Autodesk Inventor part; units mm, degrees
ref_plane "Work Plane1" through (-11.0913, 6.35, -8.8477) normal (0, -0.4472, -0.8944) x (1, 0, 0)
ref_plane "Work Plane2" through (-7.9163, 6.35, -5.6727) normal (-0.8944, -0.4472, 0) x (0, 0, -1)
ref_plane "Work Plane3" through (-7.9163, 6.35, -5.6727) normal (-0.8944, 0.4472, 0) x (0, 0, -1)
sketch "Sketch1" plane through (0, 0, 0) normal (0, 1, 0) x (-1, 0, 0)
  line L0 (11.0913, -5.6727) -> (4.7413, -5.6727)
  line L1 (4.7413, -5.6727) -> (4.7413, -12.0227)
  line L2 (4.7413, -12.0227) -> (11.0913, -12.0227)
  line L3 (11.0913, -12.0227) -> (11.0913, -5.6727)
  point P0 (0, 0)
  dimension "d0" = 6.35
  dimension "d1" = 6.35
extrude "Extrusion1" add sketch "Sketch1" along normal blind 6.35
sketch "Sketch2" plane through (0, 6.35, 0) normal (0, 1, 0) x (1, 0, 0)
  line L0 (-11.0913, 5.6727) -> (-4.7413, 5.6727)
  line L1 (-7.9163, 5.6727) -> (-7.9163, 31.288)
  line L2 (-11.0913, 12.0227) -> (-11.0913, 5.6727)
  line L3 (-11.0913, 8.8477) -> (-4.7413, 8.8477)
  line L4 (-4.7413, 5.6727) -> (-4.7413, 12.0227)
  point P0 (0, 0)
ref_plane "Work Plane1" through (-11.0913, 6.35, -8.8477) normal (0, -0.4472, -0.8944) x (1, 0, 0)
ref_plane "Work Plane2" through (-7.9163, 6.35, -5.6727) normal (-0.8944, -0.4472, 0) x (0, 0, -1)
sketch "Sketch3" plane through (-7.9163, 6.35, -5.6727) normal (-0.8944, -0.4472, 0) x (0, 0, -1)
  circle A0 centre (4.2078, 1.1693) radius 62.6047
  point P0 (-5.6727, 9.2199)
extrude "Extrusion2" cut sketch "Sketch3" against normal blind 6.35
sketch "Sketch4" plane through (-11.0913, 6.35, -8.8477) normal (0, -0.4472, -0.8944) x (1, 0, 0)
  circle A0 centre (3.6539, 12.2089) radius 78.9893
  point P0 (11.0913, 9.6364)
extrude "Extrusion3" cut sketch "Sketch4" against normal blind 6.35
ref_plane "Work Plane3" through (-7.9163, 6.35, -5.6727) normal (-0.8944, 0.4472, 0) x (0, 0, -1)
sketch "Sketch5" plane through (-7.9163, 6.35, -5.6727) normal (-0.8944, 0.4472, 0) x (0, 0, -1)
  circle A0 centre (14.7734, 12.1787) radius 25.4
  point P0 (-5.6727, 2.1393)
  dimension "d14" = 50.8
extrude "Extrusion4" cut sketch "Sketch5" along normal blind 6.35
ref_plane "Work Plane4" through (-11.0913, 6.35, -8.8477) normal (0, 0.4472, -0.8944) x (1, 0, 0)
sketch "Sketch6" plane through (-11.0913, 6.35, -8.8477) normal (0, 0.4472, -0.8944) x (1, 0, 0)
  circle A0 centre (11.0913, 15.7599) radius 33.5156
  point P0 (11.0913, 1.7228)
extrude "Extrusion5" cut sketch "Sketch6" along normal blind 6.35
properties part number "PyramidPiece-ver1-1111-2021"
Model file for the job. Use its own axes, mm. Coordinates: 2 decimals unless noted, no trailing zeros. Loops run counter-clockwise (first coordinate to the right, second up) from the corner with the lowest first, then second, coordinate; pieces in that order, holes last. Notation, with made-up numbers: (71, -29) - (128, -29) arc R11 cw to (128, -14) - close; hole circle Ø1 at (21, 38). An arc over 180 degrees is marked (long way). Answer as a JSON object with one key per item and string values. Group by question number.
(1) Probe line 1 along X through (y, z) = (2.75, -7.5); line 2 along Z through (x, y) = (-5.25, 0.5); line 3 along Y through (x, z) = (-5.25, -9.25). List the from-to ranges inside material, lowest first.
(2) Flat gauge pins, fed straight in: pin 1 (2 mm diameter, centred on x = -10, z = -8.5, fed in from +Y); pin 2 (3 mm diameter, centred on y = 3.5, z = -8.5, fed in from +X); pin 3 (1.5 mm diameter, centred on x = -8, y = 4.5, fed in from +Z). Where does each tip first touch, or does it go through?
(3) Cut at B-B (y = 4.75). Give the cut face in (x, z).
(4) Cut at A-A (z = -6.5). Give the cut face in (x, y).
Geometry says:
{
 "1": {"line 1": "x = -9.71 to -6.12", "line 2": "z = -11.77 to -5.92", "line 3": "y = 0 to 1.01"},
 "2": {"pin 1": "stops at y = 4.18", "pin 2": "stops at x = -5.74", "pin 3": "stops at z = -7.55"},
 "3": {"outline": "(-8.71, -9.65) - (-7.12, -9.65) - (-7.12, -8.05) - (-8.71, -8.05) - close"},
 "4": {"outline": "(-11.09, 0) - (-4.74, 0) - (-5.57, 1.65) - (-10.26, 1.65) - close"}
}
